from build123d import *

# Parameters (mm, degrees)
SKETCH1_R           = 15
SKETCH1_R_2         = 1.5
BOSS_EXTRUDE1_DEPTH = 4
SKETCH2_R           = 2.1
CUT_EXTRUDE1_DEPTH  = 2
SKETCH3_R           = 21.629030548
SKETCH3_R_2         = 4.1
CUT_EXTRUDE2_DEPTH  = 1.5


with BuildPart() as part:
    # Sketch1 → Boss-Extrude1 (new body)
    with BuildSketch(Plane(origin=(0, 0, 0), x_dir=(1, 0, 0), z_dir=(0, 1, 0))):
        with Locations(Location((-8.445672376, 3.816794247, 0), (0, 0, 270))):
            Circle(SKETCH1_R)
        with Locations(Location((-8.445672376, 15.816794247, 0), (0, 0, 270))):
            Circle(SKETCH1_R_2, mode=Mode.SUBTRACT)
        with Locations(Location((0.039608998, 12.302075621, 0), (0, 0, 270))):
            Circle(SKETCH1_R_2, mode=Mode.SUBTRACT)
        with Locations(Location((3.554327624, 3.816794247, 0), (0, 0, 270))):
            Circle(SKETCH1_R_2, mode=Mode.SUBTRACT)
        with Locations(Location((0.039608998, -4.668487127, 0), (0, 0, 270))):
            Circle(SKETCH1_R_2, mode=Mode.SUBTRACT)
        with Locations(Location((-8.445672376, -8.183205753, 0), (0, 0, 270))):
            Circle(SKETCH1_R_2, mode=Mode.SUBTRACT)
        with Locations(Location((-16.93095375, -4.668487127, 0), (0, 0, 270))):
            Circle(SKETCH1_R_2, mode=Mode.SUBTRACT)
        with Locations(Location((-20.445672376, 3.816794247, 0), (0, 0, 270))):
            Circle(SKETCH1_R_2, mode=Mode.SUBTRACT)
        with Locations(Location((-16.93095375, 12.302075621, 0), (0, 0, 270))):
            Circle(SKETCH1_R_2, mode=Mode.SUBTRACT)
    extrude(amount=BOSS_EXTRUDE1_DEPTH)

    # Sketch2 → Cut-Extrude1 (cut)
    with BuildSketch(Plane(origin=(0, 4, 0), x_dir=(1, 0, 0), z_dir=(0, 1, 0))):
        with Locations(Location((-8.445672376, 3.816794247, 0), (0, 0, 270))):
            Circle(SKETCH2_R)
    extrude(amount=-CUT_EXTRUDE1_DEPTH, mode=Mode.SUBTRACT)

    # Sketch3 → Cut-Extrude2 (cut)
    with BuildSketch(Plane(origin=(0, 4, 0), x_dir=(1, 0, 0), z_dir=(0, 1, 0))):
        with Locations((-8.445672376, 3.816794247)):
            Circle(SKETCH3_R)
        with Locations(Location((-8.445672376, 3.816794247, 0), (0, 0, 270))):
            Circle(SKETCH3_R_2, mode=Mode.SUBTRACT)
    extrude(amount=-CUT_EXTRUDE2_DEPTH, mode=Mode.SUBTRACT)


solid = part.part
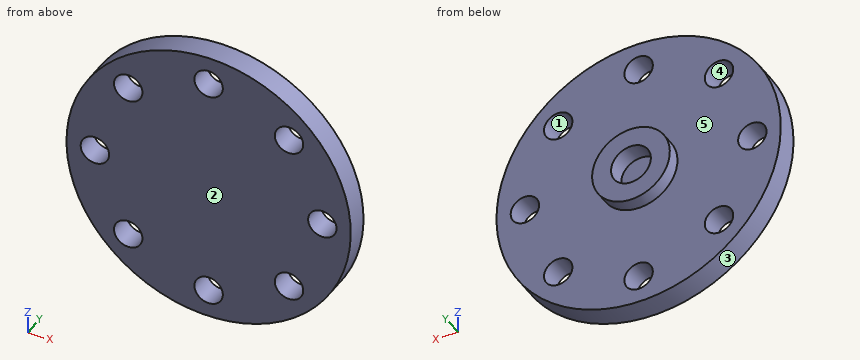
Source: CAD feature listing. Evaluate the final solid. Frame: model axes, mm. Face numbers are marked on the shaded views. A direction names the side the tool comes from. Give positions to 0.01 mm unless a question says otherwise; leave off trailing zeros. Write each loop counter-clockwise with the first axis right and the second up, starting at its lowest first coordinate (ties: lowest second). Pieces come first, ordered by that corner, then holes. Notation, with made-up numbers: (43, 0.5) -> (94, 0.5) arc R20 ccw to (94, 31.5) -> close; hole circle Ø6 at (81.5, -5). An arc over 180 degrees is marked (long way). Return JSON: item names as keys, results as strings. Group by question number.
1. Section C-C, the plane x = -19.5. Output: boundary loops of the cut face in (y, z).
2. Section B-B, the plane y = 1.5. Count the separate pieces of the cut face and the enclosed holes in it, then the cut area to 3 significant figures.
3. Access query for the marked faces 4 and 5. Directions: +Z, -Z, +X, -X, +Y, -Y. A direction counts if a zero-diameter tool reaches every point of the face in a straight line with its end or side. Return the directions, or none.
4. Mould query, pull axis Z, two halves, no side actions, for the marked faces 1, 2 and 3. Classes: +Z half, -Z half, draft (parallel to the pull), parting line (faces both ways), or undercut.
5. Section A-A, the plane z = -15.5. Output: boundary loops of the cut face in (x, y), then the cut area to 3 significant figures.
6. Material intervals for line 1 (X direction, y = 0.25, z = -5); line 2 (X direction, y = 2.85, z = -4); line 3 (X direction, y = 1.65, z = -4), sorted ascending. Write a range as from..to.
7. Section D-D, the plane z = 4.25. Output: boundary loops of the cut face in (x, y), then the cut area to 3 significant figures.
8. Pin query (flat end, axial travel): pin 1 Ø6 at (x, z) = (-4, -15.5) entering from +Y; pin 2 Ø1 at (y, z) = (3.5, -5) entering from -X. Return the tip coordinate at first contact, or that it passes through.
Determined:
{
 "1": {"outline": "(0, -13.96) -> (2.5, -13.96) -> (2.5, -4.98) -> (0, -4.98) -> close; (0, -2.65) -> (2.5, -2.65) -> (2.5, 6.32) -> (0, 6.32) -> close"},
 "2": {"separate pieces": "1", "enclosed holes": "8", "area": "650 mm2"},
 "3": {"face 4": "+Y, -Y", "face 5": "+Y"},
 "4": {"face 1": "undercut", "face 2": "draft", "face 3": "parting line"},
 "5": {"outline": "(-17.85, 0) -> (-9.91, 0) -> (-9.91, 2.5) -> (-17.85, 2.5) -> close; (-6.98, 0) -> (0.96, 0) -> (0.96, 2.5) -> (-6.98, 2.5) -> close", "area": "39.7 mm2"},
 "6": {"line 1": "x = -23.4..-21.37, -19.52..2.63, 4.48..6.51", "line 2": "x = -12.54..-10.54, -6.35..-4.35", "line 3": "x = -23.44..-21.93, -18.96..2.07, 5.04..6.55"},
 "7": {"outline": "(-21.09, 0) -> (-18.37, 0) -> (-18.37, 2.5) -> (-21.09, 2.5) -> close; (-15.49, 0) -> (-1.4, 0) -> (-1.4, 2.5) -> (-15.49, 2.5) -> close; (1.48, 0) -> (4.2, 0) -> (4.2, 2.5) -> (1.48, 2.5) -> close", "area": "48.8 mm2"},
 "8": {"pin 1": "stops at y = 2.5", "pin 2": "stops at x = -12.49"}
}
